The model under review builds one solid part; all positions refer to its coordinate system, in mm. A direction names the side the tool comes from. Round coordinates to 2 decimals unless told otherwise and drop trailing zeros. Loops run counter-clockwise (first coordinate to the right, second up) from the corner with the lowest first, then second, coordinate; pieces in that order, holes last. Notation, with made-up numbers: (-4.5, -7.75) -> (33.5, -7.75) arc R24 ccw to (33.5, 10.25) -> close; hole circle Ø5 at (15, 88.25). An arc over 180 degrees is marked (long way). Use CSV: the item, a comma, the result in double quotes. Start each with the question number.
```python
from build123d import *

# Parameters (mm, degrees)
SKETCH1_W                                            = 190
SKETCH1_H                                            = 32
BOSS_EXTRUDE1_DEPTH                                  = 16
CHAMFER1_SIZE                                        = 2
SKETCH2_W                                            = 25
SKETCH2_H                                            = 4
CUT_EXTRUDE1_DEPTH                                   = 33
M12_TAPPED_HOLE1_D                                   = 10.2
M12_TAPPED_HOLE1_DEPTH                               = 24
M12_TAPPED_HOLE1_CSINK_D                             = 12.005
M12_TAPPED_HOLE1_CSINK_ANGLE                         = 90
M12_TAPPED_HOLE1_TIP                                 = 3.064389157
M4_TAPPED_HOLE2_D                                    = 3.3
M4_TAPPED_HOLE2_DEPTH                                = 11.5
M4_TAPPED_HOLE2_CSINK_D                              = 4.05
M4_TAPPED_HOLE2_CSINK_ANGLE                          = 90
M4_TAPPED_HOLE2_TIP                                  = 0.991420021
CSK_FOR_M10_COUNTERSUNK_FLAT_HEAD_SCREW1_D           = 6.5
CSK_FOR_M10_COUNTERSUNK_FLAT_HEAD_SCREW1_CSINK_D     = 13
CSK_FOR_M10_COUNTERSUNK_FLAT_HEAD_SCREW1_CSINK_ANGLE = 90
SKETCH16_R                                           = 3
CUT_EXTRUDE2_DEPTH                                   = 33
CSK_FOR_M4_COUNTERSUNK_FLAT_HEAD_SCREW1_D            = 1.5
CSK_FOR_M4_COUNTERSUNK_FLAT_HEAD_SCREW1_DEPTH        = 10
CSK_FOR_M4_COUNTERSUNK_FLAT_HEAD_SCREW1_CSINK_D      = 4
CSK_FOR_M4_COUNTERSUNK_FLAT_HEAD_SCREW1_CSINK_ANGLE  = 90
CSK_FOR_M4_COUNTERSUNK_FLAT_HEAD_SCREW1_TIP          = 0.450645464
M4_TAPPED_HOLE3_D                                    = 3.3
M4_TAPPED_HOLE3_DEPTH                                = 16
M4_TAPPED_HOLE3_CSINK_D                              = 4.05
M4_TAPPED_HOLE3_CSINK_ANGLE                          = 90
M4_TAPPED_HOLE3_TIP                                  = 0.991420021
SKETCH24_R                                           = 3
CUT_EXTRUDE4_DEPTH                                   = 33


with BuildPart() as part:
    # Sketch1 → Boss-Extrude1 (new body, symmetric)
    with BuildSketch(Plane.XY):
        Rectangle(SKETCH1_W, SKETCH1_H)
    extrude(amount=BOSS_EXTRUDE1_DEPTH, both=True)

    # Chamfer1
    chamfer1_edges = [part.edges().sort_by_distance(p)[0] for p in [
        (-95, 0, 16),
        (95, 0, 16),
        (-95, 0, -16),
    ]]
    chamfer(chamfer1_edges, length=CHAMFER1_SIZE)

    # Sketch2 → Cut-Extrude1 (cut, through all)
    with BuildSketch(Plane(origin=(0, 16, 0), x_dir=(1, 0, 0), z_dir=(0, 1, 0))):
        with Locations((79.5, 14)):
            Rectangle(SKETCH2_W, SKETCH2_H)
    extrude(amount=-CUT_EXTRUDE1_DEPTH, mode=Mode.SUBTRACT)

    # M12 Tapped Hole1
    with Locations(Plane(origin=(0, 16, 0), x_dir=(1, 0, 0), z_dir=(0, 1, 0))):
        with Locations((-63, 0), (11, 0)):
            CounterSinkHole(M12_TAPPED_HOLE1_D / 2, M12_TAPPED_HOLE1_CSINK_D / 2, depth=M12_TAPPED_HOLE1_DEPTH, counter_sink_angle=M12_TAPPED_HOLE1_CSINK_ANGLE)
            with Locations((0, 0, -(M12_TAPPED_HOLE1_DEPTH + M12_TAPPED_HOLE1_TIP / 2))):  # 118° drill point
                Cone(0, M12_TAPPED_HOLE1_D / 2, M12_TAPPED_HOLE1_TIP, mode=Mode.SUBTRACT)

    # M4 Tapped Hole2
    with Locations(Plane(origin=(-63, 4, 16), x_dir=(1, 0, 0), z_dir=(0, 0, 1))):
        with Locations((0, 0), (74, 0)):
            CounterSinkHole(M4_TAPPED_HOLE2_D / 2, M4_TAPPED_HOLE2_CSINK_D / 2, depth=M4_TAPPED_HOLE2_DEPTH, counter_sink_angle=M4_TAPPED_HOLE2_CSINK_ANGLE)
            with Locations((0, 0, -(M4_TAPPED_HOLE2_DEPTH + M4_TAPPED_HOLE2_TIP / 2))):  # 118° drill point
                Cone(0, M4_TAPPED_HOLE2_D / 2, M4_TAPPED_HOLE2_TIP, mode=Mode.SUBTRACT)

    # CSK for M10 Countersunk Flat Head Screw1 (through all)
    with Locations(Plane.XY.offset(16)):
        with Locations((79.5, 4)):
            CounterSinkHole(CSK_FOR_M10_COUNTERSUNK_FLAT_HEAD_SCREW1_D / 2, CSK_FOR_M10_COUNTERSUNK_FLAT_HEAD_SCREW1_CSINK_D / 2, counter_sink_angle=CSK_FOR_M10_COUNTERSUNK_FLAT_HEAD_SCREW1_CSINK_ANGLE)

    # Sketch16 → Cut-Extrude2 (cut, through all)
    with BuildSketch(Plane.XY.offset(16)):
        with Locations((-87, 6)):
            Circle(SKETCH16_R)
    extrude(amount=-CUT_EXTRUDE2_DEPTH, mode=Mode.SUBTRACT)

    # CSK for M4 Countersunk Flat Head Screw1
    with Locations(Plane(origin=(0, 16, 0), x_dir=(1, 0, 0), z_dir=(0, 1, 0))):
        with Locations((-87, 0)):
            CounterSinkHole(CSK_FOR_M4_COUNTERSUNK_FLAT_HEAD_SCREW1_D / 2, CSK_FOR_M4_COUNTERSUNK_FLAT_HEAD_SCREW1_CSINK_D / 2, depth=CSK_FOR_M4_COUNTERSUNK_FLAT_HEAD_SCREW1_DEPTH, counter_sink_angle=CSK_FOR_M4_COUNTERSUNK_FLAT_HEAD_SCREW1_CSINK_ANGLE)
            with Locations((0, 0, -(CSK_FOR_M4_COUNTERSUNK_FLAT_HEAD_SCREW1_DEPTH + CSK_FOR_M4_COUNTERSUNK_FLAT_HEAD_SCREW1_TIP / 2))):  # 118° drill point
                Cone(0, CSK_FOR_M4_COUNTERSUNK_FLAT_HEAD_SCREW1_D / 2, CSK_FOR_M4_COUNTERSUNK_FLAT_HEAD_SCREW1_TIP, mode=Mode.SUBTRACT)

    # M4 Tapped Hole3
    with Locations(Plane(origin=(0, 16, 0), x_dir=(1, 0, 0), z_dir=(0, 1, 0))):
        with Locations((-43, 0)):
            CounterSinkHole(M4_TAPPED_HOLE3_D / 2, M4_TAPPED_HOLE3_CSINK_D / 2, depth=M4_TAPPED_HOLE3_DEPTH, counter_sink_angle=M4_TAPPED_HOLE3_CSINK_ANGLE)
            with Locations((0, 0, -(M4_TAPPED_HOLE3_DEPTH + M4_TAPPED_HOLE3_TIP / 2))):  # 118° drill point
                Cone(0, M4_TAPPED_HOLE3_D / 2, M4_TAPPED_HOLE3_TIP, mode=Mode.SUBTRACT)

    # Sketch24 → Cut-Extrude4 (cut, through all)
    with BuildSketch(Plane(origin=(0, 16, 0), x_dir=(1, 0, 0), z_dir=(0, 1, 0))):
        with Locations((-37, 10)):
            Circle(SKETCH24_R)
        with Locations((37, 10)):
            Circle(SKETCH24_R)
    extrude(amount=-CUT_EXTRUDE4_DEPTH, mode=Mode.SUBTRACT)


solid = part.part
```
1. Take a section at B-B, the plane x = 79.5. Give the boundary of the cut face in (y, z), then the cut area to 3 significant figures.
2. For line 1 along X through (y, z) = (8, -0.5); line 2 along X through (y, z) = (1, 3); line 3 along Z through (x, y) = (37, 6.5), list the stretches that pass through material, from the lowest coordinate up. Write a range as from..to.
3. Take a section at A-A, the plane z = -10. Give the boundary of the cut face in (x, y).
4. For faces 5 (the face through (-62, 3, -5)), 6 (the face through (67, 0, -14)), 7 (the face through (-61.35, 4.07, 10.15)), list the 3-axis set-ups (+Z, -Z, +X, -X, +Y, -Y) from which the entire face can be reached by the end or side of a thin tool; tool diameter is ignored.
5. Clearance check with flat-ended pins moving along their axes: P1, Ø2, axis at x = -87, z = 0, coming from the +Y side; P2, Ø7.5, axis at x = 76, y = -1.5, coming from the -Z side; P3, Ø3, axis at x = -43, z = 0, coming from the +Y side. State where each tip first meets the part, or that it passes through.
6. The part is to be moulded in two halves that separate along X. For faces 1 (the face through (-95, 0, 0)), 2 (the face through (-88, 15, 0)), 3 (the face through (-1, 16, 0)), 4 (the face through (82.747, 4.143, 0.202)), say which applies: pulls with the +X half, pulls with the -X half, needs draft (parallel to the pull), parting line crosses it, or undercut.
Results:
1,outline,"(-16, -12) -> (0.75, -12) -> (0.75, 12.75) -> (-2.5, 16) -> (-16, 16) -> close; (7.25, -12) -> (16, -12) -> (16, 16) -> (10.5, 16) -> (7.25, 12.75) -> close"
1,area,"703 mm²"
2,line 1,"-95..-89.24, -84.76..-68.08, -57.92..-44.57, -41.43..5.92, 16.08..95"
2,line 2,"-95..-67.12, -58.88..6.88, 15.12..78.25, 80.75..95"
2,line 3,"-16..-13, -7..16"
3,outline,"(-95, -16) -> (-40, -16) -> (-40, 16) -> (-95, 16) -> close; (-34, -16) -> (34, -16) -> (34, 16) -> (-34, 16) -> close; (40, -16) -> (95, -16) -> (95, 16) -> (40, 16) -> close; hole circle Ø6 at (-87, 6); hole circle Ø6.5 at (79.5, 4)"
4,face 5,"+Y"
4,face 6,"-Z, +Y, -Y"
4,face 7,"+Z"
5,P1,"y = 15"
5,P2,"z = -12"
5,P3,"y = -0.09"
6,face 1,"pulls with the -X half"
6,face 2,"undercut"
6,face 3,"needs draft"
6,face 4,"undercut"
